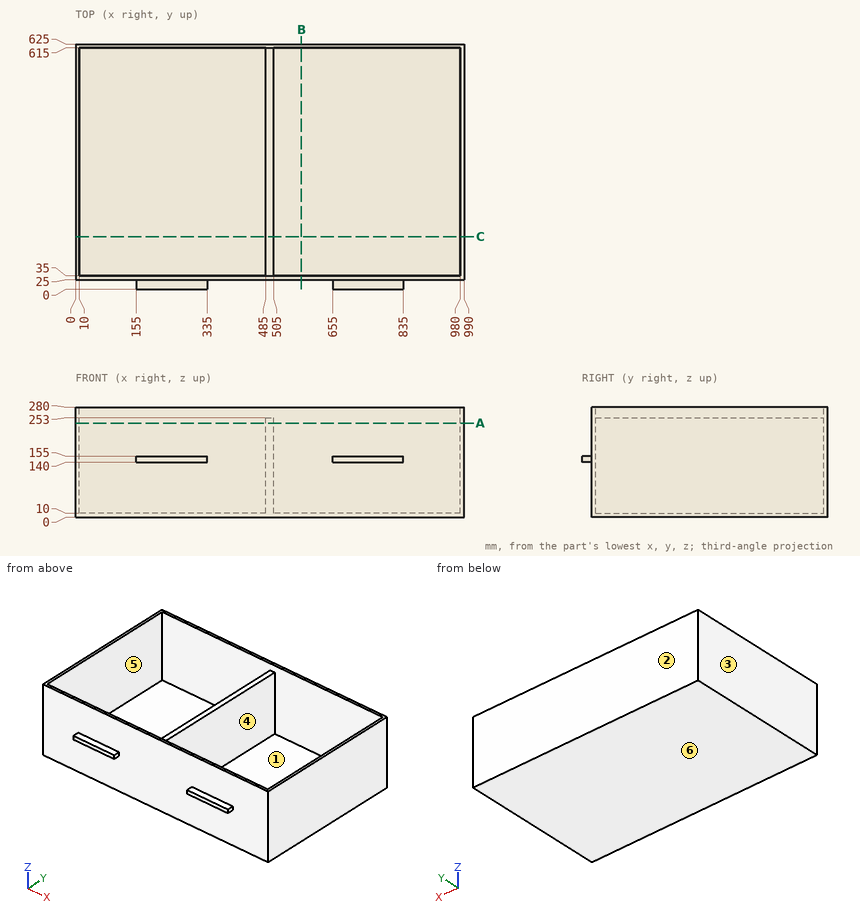
Geometry check sheet. Reference: drawing and pictorial views, mm from the part's lowest x, y, z. A direction names the side the tool comes from. Round coordinates to 2 decimals unless told otherwise and drop trailing zeros. Order: outer loops, then holes, each group sorted by start corner. A loop starts at its lowest first (then second) coordinate and runs counter-clockwise, first axis right, second up. Notation, with made-up numbers: M -0.5,53 L 40.5,53 A23 ccw 40.5,81 Z; hole C 27.25,40.5 d10. An arc over 180 degrees is marked long. Answer in a Markdown table with one row per item.
(1) Draft check along X on the marked faces 1, 2, 3 and 4. Enter one of: released by +X, released by -X, zero draft, split by the parting line, or undercut.
Responses:
| item | result |
|---|---|
| face 1 | undercut |
| face 2 | zero draft |
| face 3 | released by -X |
| face 4 | undercut |
(2) Sectioned sample at B-B, the plane x = 575.5. Record the cut outline in (y, z).
Responses:
| item | result |
|---|---|
| outline | M 25,0 L 625,0 L 625,280 L 615,280 L 615,10 L 35,10 L 35,280 L 25,280 Z |
(3) Sectioned sample at A-A, the plane z = 240. Record the cut outline in (x, y), and give its area (3 significant figures).
Responses:
| item | result |
|---|---|
| outline | M 0,25 L 990,25 L 990,625 L 0,625 Z; hole M 10,35 L 485,35 L 485,615 L 10,615 Z; hole M 505,35 L 980,35 L 980,615 L 505,615 Z |
| area | 43,000 mm² |
(4) Tool access check on the marked faces 5 and 6. Record the directions out of +Z, -Z, +X, -X, +Y, -Y that give a thin tool (end or side, any length) a straight path to the whole face; none if there is none.
Responses:
| item | result |
|---|---|
| face 5 | +Z |
| face 6 | -Z, +X, -X, +Y, -Y |
(5) Sectioned sample at C-C, the plane y = 134. Record the cut outline in (x, z), and give its area (3 significant figures).
Responses:
| item | result |
|---|---|
| outline | M 0,0 L 990,0 L 990,280 L 980,280 L 980,10 L 505,10 L 505,253 L 485,253 L 485,10 L 10,10 L 10,280 L 0,280 Z |
| area | 20,200 mm² |
(6) Scan lines: probe 1 along X at (y, z) = (144.5, 60.5); probe 2 along Y at (x, z) = (590, 33); probe 3 along X at (y, z) = (111.5, 264). Record each from-to range of solid material in increasing order. Write a range as from..to.
Responses:
| item | result |
|---|---|
| probe 1 | x = 0..10, 485..505, 980..990 |
| probe 2 | y = 25..35, 615..625 |
| probe 3 | x = 0..10, 980..990 |
(7) Go/stop test with flat-tipped pins: P1, Ø16.5, axis at y = 9, z = 149, coming from the -X side; P2, Ø7.5, axis at x = 717.5, y = 15.5, coming from the -Z side; P3, Ø12, axis at y = 6.5, z = 150.5, coming from the +X side. Record where each tip stops, or that it passes through.
Responses:
| item | result |
|---|---|
| P1 | stops at x = 155 |
| P2 | stops at z = 140 |
| P3 | stops at x = 835 |
